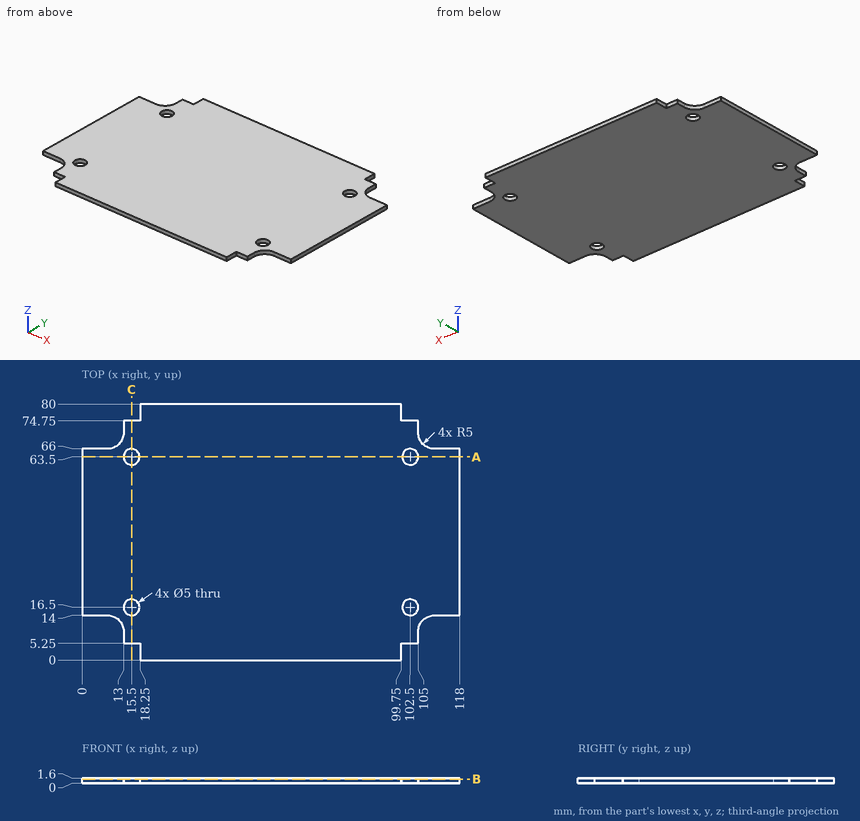
Design review of the part shown in the three views and the two pictorial views. Dimensions are in mm from the part's minimum x, y and z. Round coordinates to 2 decimals unless told otherwise and drop trailing zeros. Write each loop counter-clockwise with the first axis right and the second up, starting at its lowest first coordinate (ties: lowest second). Pieces come first, ordered by that corner, then holes. Notation, with made-up numbers: (42.5, -39) - (95.5, -39) arc R24 ccw to (95.5, -19) - close; hole circle Ø4 at (-35, 43.5). An arc over 180 degrees is marked (long way). Return JSON: item names as keys, results as strings. Group by question number.
Item 1: We need section C-C on x = 15.5. Write out the cut boundary in (y, z), and give its area (3 significant figures).
Item 2: We need section B-B on z = 1.3. Write out the cut boundary in (x, y).
Item 3: Insertion check: P1, Ø0.5, axis at x = 16.5, z = 0.5, coming from the +Y side; P2, Ø4, axis at x = 15.5, y = 63.5, coming from the -Z side; P3, Ø0.8, axis at x = 3.5, z = 1, coming from the -Y side; P4, Ø0.8, axis at x = 5.5, z = 0.5, coming from the +Y side. Each pin has a flat end and moves straight along its axis. Give the tip position at first contact, or say it passes through.
Item 4: For probe 1 along Y at (x, z) = (102.5, 0.6); probe 2 along X at (y, z) = (18, 0.3); probe 3 along X at (y, z) = (62.5, 1.15), list the stretches that pass through material, from the lowest coordinate up. Write a range as [from, to].
Item 5: We need section A-A on y = 63.5. Write out the cut boundary in (x, z), and give its area (3 significant figures).
Model answer:
{
 "1": {"outline": "(5.25, 0) - (14, 0) - (14, 1.6) - (5.25, 1.6) - close; (19, 0) - (61, 0) - (61, 1.6) - (19, 1.6) - close; (66, 0) - (74.75, 0) - (74.75, 1.6) - (66, 1.6) - close", "area": "95.2 mm²"},
 "2": {"outline": "(0, 14) - (8, 14) arc R5 cw to (13, 9) - (13, 5.25) - (18.25, 5.25) - (18.25, 0) - (99.75, 0) - (99.75, 5.25) - (105, 5.25) - (105, 9) arc R5 cw to (110, 14) - (118, 14) - (118, 66) - (110, 66) arc R5 cw to (105, 71) - (105, 74.75) - (99.75, 74.75) - (99.75, 80) - (18.25, 80) - (18.25, 74.75) - (13, 74.75) - (13, 71) arc R5 cw to (8, 66) - (0, 66) - close; hole circle Ø5 at (15.5, 16.5); hole circle Ø5 at (15.5, 63.5); hole circle Ø5 at (102.5, 16.5); hole circle Ø5 at (102.5, 63.5)"},
 "3": {"P1": "stops at y = 74.75", "P2": "passes through", "P3": "stops at y = 14", "P4": "stops at y = 66"},
 "4": {"probe 1": "y = [5.25, 14], [19, 61], [66, 74.75]", "probe 2": "x = [0, 13.5], [17.5, 100.5], [104.5, 118]", "probe 3": "x = [0, 13.21], [17.79, 100.21], [104.79, 118]"},
 "5": {"outline": "(0, 0) - (13, 0) - (13, 1.6) - (0, 1.6) - close; (18, 0) - (100, 0) - (100, 1.6) - (18, 1.6) - close; (105, 0) - (118, 0) - (118, 1.6) - (105, 1.6) - close", "area": "173 mm²"}
}
